Part print with two shaded views. Sizes in mm from the minimum x, y, z corner. Give positions to 0.01 mm unless a question says otherwise; leave off trailing zeros. Write each loop counter-clockwise with the first axis right and the second up, starting at its lowest first coordinate (ties: lowest second). Pieces come first, ordered by that corner, then holes.
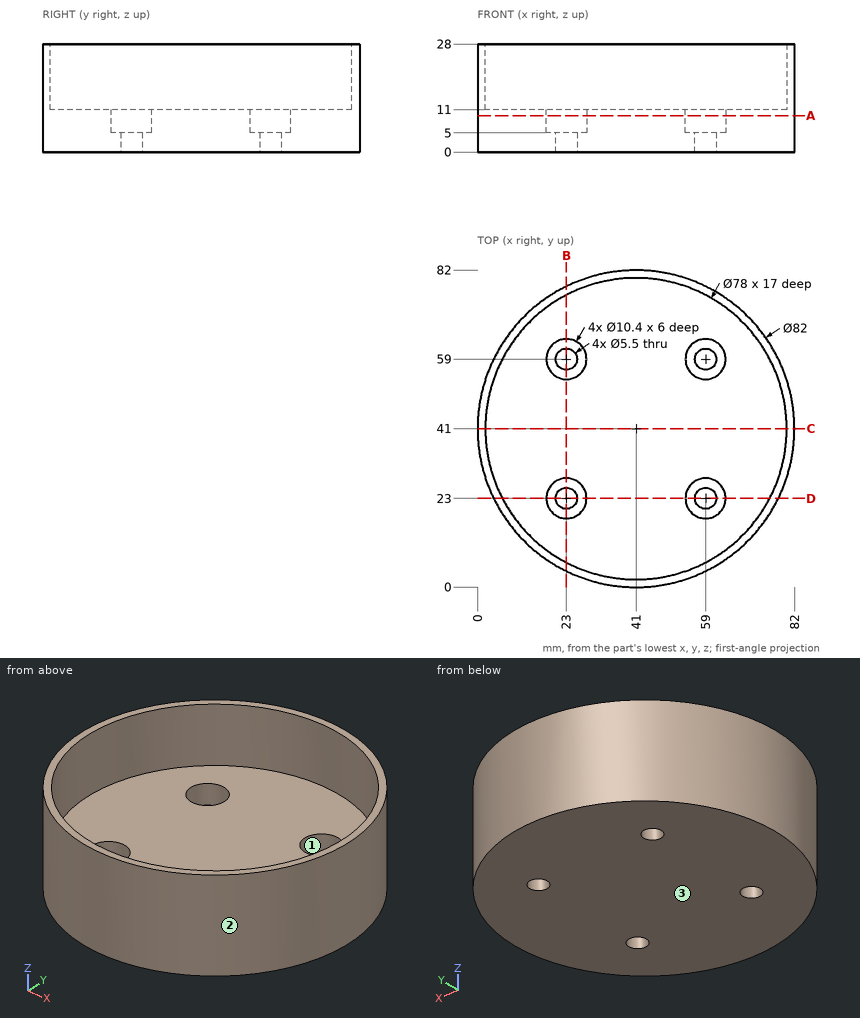
1) Mould opens along X. For the marked faces 1, 2 and 3 say: +X half, -X half, draft (parallel to the pull), parting line (faces both ways), or undercut.
Check result:
face 1: undercut
face 2: parting line
face 3: draft
2) Saw through at A-A (z = 9.5). Write the cut outline in (x, y).
Check result:
outline: circle Ø82 at (41, 41); hole circle Ø10.4 at (23, 23); hole circle Ø10.4 at (23, 59); hole circle Ø10.4 at (59, 23); hole circle Ø10.4 at (59, 59)
3) Flat gauge pins, fed straight in: P1, Ø6, axis at x = 36, z = 15.5, coming from the +Y side; P2, Ø6.5, axis at x = 23, y = 23, coming from the +Z side; P3, Ø1, axis at y = 58.5, z = 17, coming from the +X side. Where does each tip first touch, or does it go through?
Check result:
P1: stops at y = 81.95
P2: stops at z = 5
P3: stops at x = 78.31
4) Drill centre lines: L1, parallel to Y at x = 41, z = 16; L2, parallel to Y at x = 59, z = 7.75; L3, parallel to Y at x = 26, z = 10. Where is each one in solid material? Low to high.
Check result:
L1: y = 0 to 2, 80 to 82
L2: y = 4.16 to 17.8, 28.2 to 53.8, 64.2 to 77.84
L3: y = 2.84 to 18.75, 27.25 to 54.75, 63.25 to 79.16
5) Saw through at B-B (x = 23). Write the cut outline in (y, z), and give its area (3 significant figures).
Check result:
outline: (4.16, 0) - (20.25, 0) - (20.25, 5) - (17.8, 5) - (17.8, 11) - (6.4, 11) - (6.4, 28) - (4.16, 28) - close; (25.75, 0) - (56.25, 0) - (56.25, 5) - (53.8, 5) - (53.8, 11) - (28.2, 11) - (28.2, 5) - (25.75, 5) - close; (61.75, 0) - (77.84, 0) - (77.84, 28) - (75.6, 28) - (75.6, 11) - (64.2, 11) - (64.2, 5) - (61.75, 5) - close
area: 707 mm2
6) Saw through at C-C (y = 41). Write the cut outline in (x, z).
Check result:
outline: (0, 0) - (82, 0) - (82, 28) - (80, 28) - (80, 11) - (2, 11) - (2, 28) - (0, 28) - close
